Here's how the part is built. I have some questions about the finished solid (model axes, mm). Face numbers are marked on the shaded views. A direction names the side the tool comes from. Coordinates: 2 decimals unless noted, no trailing zeros. Write each loop counter-clockwise with the first axis right and the second up, starting at its lowest first coordinate (ties: lowest second). Pieces come first, ordered by that corner, then holes. Notation, with made-up numbers: (-39.75, -17.75) -> (-30.75, -17.75) arc R8 cw to (-30.75, -3.75) -> close; hole circle Ø2 at (-13.75, 49.5). An arc over 180 degrees is marked (long way). Put each result on its own line as item: value.
```python
from build123d import *

# Parameters (mm, degrees)
SKETCH_1_R      = 2.5
EXTRUDE_1_DEPTH = 2


with BuildPart() as part:
    # 스케치1 → 보스-돌출1 (new body)
    with BuildSketch(Plane.XY):
        with BuildLine():
            Line((20.887065526, -4.904042543), (17.65515334, -8.287321674))
            ThreePointArc((17.65515334, -8.287321674), (14.119619434, -9.751787768), (12.65515334, -13.287321674))
            Line((12.65515334, -13.287321674), (12.65515334, -39.724999499))
            Line((12.65515334, -39.724999499), (15.15515334, -39.724999499))
            Line((15.15515334, -39.724999499), (15.15515334, -43.161796007))
            ThreePointArc((15.15515334, -43.161796007), (18.953651475, -43.238083254), (22.731294666, -42.833336733))
            Line((22.731294666, -42.833336733), (22.731294666, -44.249079054))
            Line((22.731294666, -44.249079054), (25.163405743, -44.249079054))
            ThreePointArc((25.163405743, -44.249079054), (27.284726086, -43.370399397), (28.163405743, -41.249079054))
            Line((28.163405743, -41.249079054), (28.163405743, -39.724999499))
            Line((28.163405743, -39.724999499), (25.906714003, -39.724999499))
            Line((25.906714003, -39.724999499), (23.650022264, -39.724999499))
            Line((23.650022264, -39.724999499), (23.650022264, -18.287321674))
            Line((23.650022264, -18.287321674), (37.65515334, -18.287321674))
            ThreePointArc((37.65515334, -18.287321674), (41.190687246, -16.82285558), (42.65515334, -13.287321674))
            Line((42.65515334, -13.287321674), (42.65515334, -9.191405084))
            Line((42.65515334, -9.191405084), (41.15515334, -9.191405084))
            Line((41.15515334, -9.191405084), (41.15515334, -10.336593208))
            Line((41.15515334, -10.336593208), (37.25515334, -10.336593208))
            Line((37.25515334, -10.336593208), (37.25515334, -8.508126005))
            ThreePointArc((37.25515334, -8.508126005), (37.192620725, -8.342729573), (37.036305504, -8.260074513))
            ThreePointArc((37.036305504, -8.260074513), (28.894559444, -6.905069462), (20.887065526, -4.904042543))
        make_face()
        with Locations((17.65515334, -13.287321674)):
            Circle(SKETCH_1_R, mode=Mode.SUBTRACT)
    extrude(amount=EXTRUDE_1_DEPTH)


solid = part.part
```
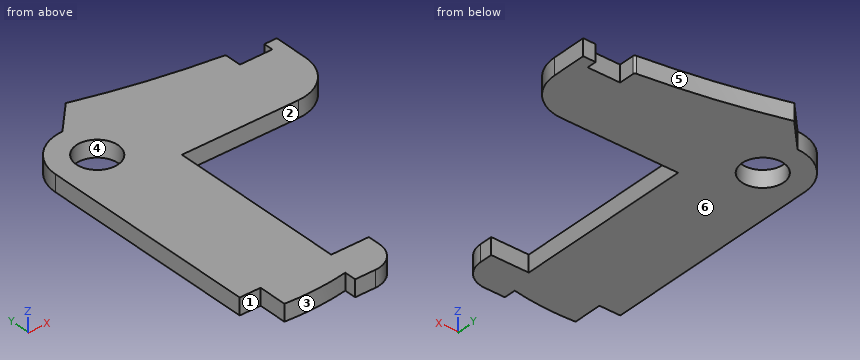
Item 1: Imagine slicing it at C-C on y = -29. Write out the boundary of the cut face in (x, z), then the cut area to 3 significant figures.
Output:
outline: (12.66, 0) -> (23.65, 0) -> (23.65, 2) -> (12.66, 2) -> close
area: 22.0 mm²
Item 2: Imagine slicing it at D-D on x = 22. Write out the boundary of the cut face in (y, z), then the cut area to 3 significant figures.
Output:
outline: (-42.95, 0) -> (-5.22, 0) -> (-5.22, 2) -> (-42.95, 2) -> close
area: 75.5 mm²
Item 3: Imagine slicing it at A-A on z = 0.75. Write out the boundary of the cut face in (x, y) (3 decimals).
Output:
outline: (12.655, -39.725) -> (15.155, -39.725) -> (15.155, -43.162) arc R29.979 ccw to (22.731, -42.833) -> (22.731, -44.249) -> (25.163, -44.249) arc R3 ccw to (28.163, -41.249) -> (28.163, -39.725) -> (23.65, -39.725) -> (23.65, -18.287) -> (37.655, -18.287) arc R5 ccw to (42.655, -13.287) -> (42.655, -9.191) -> (41.155, -9.191) -> (41.155, -10.337) -> (37.255, -10.337) -> (37.255, -8.508) arc R0.25 ccw to (37.036, -8.26) arc R103.246 cw to (20.887, -4.904) -> (17.655, -8.287) arc R5 ccw to (12.655, -13.287) -> close; hole circle Ø5 at (17.655, -13.287)
Item 4: For P1, Ø0.9, axis at y = -10, z = 1.5, coming from the -X side; P2, Ø1.2, axis at x = 41.5, z = 0.5, coming from the +Y side; P3, Ø0.6, axis at y = -41, z = 1, coming from the -X side, each with a flat end and sliding along its axis, tell me the tip position at first contact or that it passes through.
Output:
P1: stops at x = 13.54
P2: stops at y = -9.19
P3: stops at x = 15.16
Item 5: Please list where these lines run through material, in increasing order: line 1 along Y through (x, z) = (19, 1.15); line 2 along X through (y, z) = (-15.5, 0.7); line 3 along X through (y, z) = (-14.5, 1.8). Write a range as from..to.
Output:
line 1: y = -43.24..-15.39, -11.18..-6.88
line 2: x = 12.66..16.49, 18.82..42.14
line 3: x = 12.66..15.47, 19.84..42.51
Item 6: Imagine slicing it at B-B on x = 19. Write out the boundary of the cut face in (y, z), then the cut area to 3 significant figures.
Output:
outline: (-43.24, 0) -> (-15.39, 0) -> (-15.39, 2) -> (-43.24, 2) -> close; (-11.18, 0) -> (-6.88, 0) -> (-6.88, 2) -> (-11.18, 2) -> close
area: 64.3 mm²
Item 7: If we mould it in two halves opening along X, with no side actions, what happens to the marked faces 4, 5 and 6? For each: released by +X, released by -X, zero draft, split by the parting line, or undercut.
Output:
face 4: undercut
face 5: released by +X
face 6: zero draft
Item 8: Which directions (+Z, -Z, +X, -X, +Y, -Y) give clear straight access to the entire face, cutting with the end or side of a thin tool? Please do the marked faces 1, 2 and 3.
Output:
face 1: +Z, -Z, -X, -Y
face 2: +Z, -Z, +X
face 3: +Z, -Z, -Y
